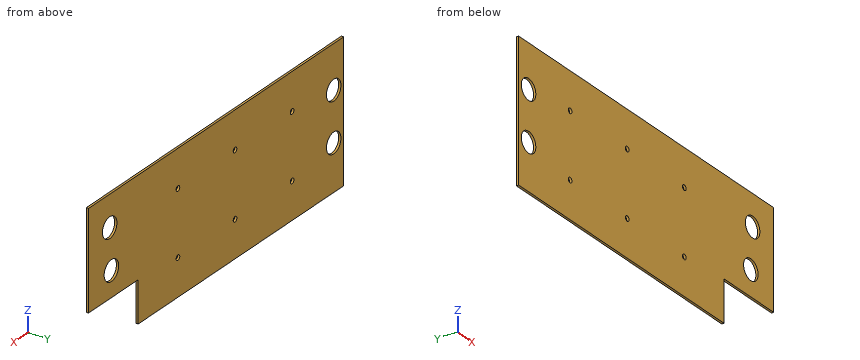
```python
from build123d import *

# Parameters (mm, degrees)
BOSS_EXTRUDE1_DEPTH     = 3.5
CUT_EXTRUDE1_DEPTH      = 599.744260933
CUT_EXTRUDE1_DEPTH_BACK = 599.744260933
SKETCH2_R               = 4
SKETCH3_R               = 15.875
CUT_EXTRUDE2_DEPTH      = 10


with BuildPart() as part:
    # Sketch1 → Boss-Extrude1 (new body)
    with BuildSketch(Plane(origin=(0, 0, 0), x_dir=(1, 0, 0), z_dir=(0, 1, 0))):
        Polygon((0, 0), (0, 215), (450, 215), (450, 151), (558.8, 151), (558.8, 0), align=None)
    extrude(amount=BOSS_EXTRUDE1_DEPTH)

    # Sketch2 → Cut-Extrude1 (cut, two sides: drawn at the far end of the back side and taken through both)
    with BuildSketch(Plane(origin=(0, 3.5, 0), x_dir=(1, 0, 0), z_dir=(0, 1, 0)).offset(-CUT_EXTRUDE1_DEPTH_BACK)):
        with Locations(Location((113, 157.85, 0), (0, 0, 270))):
            Circle(SKETCH2_R)
        with Locations(Location((238, 157.85, 0), (0, 0, 270))):
            Circle(SKETCH2_R)
        with Locations(Location((363, 157.85, 0), (0, 0, 270))):
            Circle(SKETCH2_R)
        with Locations(Location((363, 57.85, 0), (0, 0, 270))):
            Circle(SKETCH2_R)
        with Locations(Location((238, 57.85, 0), (0, 0, 270))):
            Circle(SKETCH2_R)
        with Locations(Location((113, 57.85, 0), (0, 0, 270))):
            Circle(SKETCH2_R)
    extrude(amount=CUT_EXTRUDE1_DEPTH + CUT_EXTRUDE1_DEPTH_BACK, mode=Mode.SUBTRACT)

    # Sketch3 → Cut-Extrude2 (cut)
    with BuildSketch(Plane(origin=(0, 3.5, 0), x_dir=(1, 0, 0), z_dir=(0, 1, 0))):
        with Locations(Location((21.977158482, 143.521297983, 0), (0, 0, 270))):
            Circle(SKETCH3_R)
        with Locations(Location((22.025, 67.321313002, 0), (0, 0, 270))):
            Circle(SKETCH3_R)
        with Locations(Location((512.5174446, 48.349661731, 0), (0, 0, 270))):
            Circle(SKETCH3_R)
        with Locations(Location((508.667649246, 111.732854107, 0), (0, 0, 270))):
            Circle(SKETCH3_R)
    extrude(amount=-CUT_EXTRUDE2_DEPTH, mode=Mode.SUBTRACT)


solid = part.part
```
Source: CAD feature listing. Evaluate the final solid. Frame: model axes, mm. Coordinates: 2 decimals unless noted, no trailing zeros. Write each loop counter-clockwise with the first axis right and the second up, starting at its lowest first coordinate (ties: lowest second). Pieces come first, ordered by that corner, then holes. Notation, with made-up numbers: (-24, -6) -> (-7, -6) arc R13 ccw to (-7, 19) -> close; hole circle Ø10 at (38.5, -20.5). An arc over 180 degrees is marked (long way). Return JSON: item names as keys, results as strings. Group by question number.
1) Section query A-A, the plane z = -116.5. Return loops of the section in (x, y), plus the area to 3 significant figures.
2) Section query C-C, the plane x = 483. Return loops of the section in (y, z).
3) Ray query, line 1 along Z through (x, y) = (363, 1.95); line 2 along X through (y, z) = (2.3, -56); line 3 along X through (y, z) = (2.4, -157.85). Return the intervals inside material, ascending.
4) Contact query for flat-ended pins moving along their axis: P1, Ø2, axis at x = 280, z = -83.5, coming from the -Y side; P2, Ø6.5, axis at x = 113, z = -157.85, coming from the +Y side; P3, Ø1, axis at x = 505, y = 1, coming from the -Z side; P4, Ø1.8, axis at y = 1, z = -182.5, coming from the +X side. Output: stop coordinate, or through.
5) Section query D-D, the plane z = -189. Return loops of the section in (x, y), plus the area to 4 significant figures.
6) Section query B-B, the plane y = 2.4. State how many separate pieces and enclosed holes the cut face has, plus the area to 3 significant figures.
From the geometry:
{
 "1": {"outline": "(0, 0) -> (493.53, 0) -> (493.53, 3.5) -> (0, 3.5) -> close; (523.81, 0) -> (558.8, 0) -> (558.8, 3.5) -> (523.81, 3.5) -> close", "area": "1,850 mm²"},
 "2": {"outline": "(0, -151) -> (3.5, -151) -> (3.5, 0) -> (0, 0) -> close"},
 "3": {"line 1": "-215 to -161.85, -153.85 to -61.85, -53.85 to 0", "line 2": "0 to 10.9, 33.15 to 109.45, 116.55 to 234.45, 241.55 to 359.45, 366.55 to 498.61, 526.43 to 558.8", "line 3": "0 to 15.14, 28.81 to 109, 117 to 234, 242 to 359, 367 to 450"},
 "4": {"P1": "y = 0", "P2": "through", "P3": "z = -151", "P4": "x = 450"},
 "5": {"outline": "(0, 0) -> (450, 0) -> (450, 3.5) -> (0, 3.5) -> close", "area": "1,575 mm²"},
 "6": {"separate pieces": "1", "enclosed holes": "10", "area": "110,000 mm²"}
}
